Model file for the job. Use its own axes, mm. A direction names the side the tool comes from. Coordinates: 2 decimals unless noted, no trailing zeros. Write each loop counter-clockwise with the first axis right and the second up, starting at its lowest first coordinate (ties: lowest second). Pieces come first, ordered by that corner, then holes. Notation, with made-up numbers: M -37.5,-12 L -24.5,-12 A22 cw -24.5,25 Z; hole C 15,-16.5 d5. An arc over 180 degrees is marked long. Put each result on its own line as item: value. Start each with the question number.
Q1. Drill centre lines: line 1 along Y through (x, z) = (12.5, 4.7); line 2 along Y through (x, z) = (3.5, 5.55); line 3 along Z through (x, y) = (35.5, 0.25). Where is each one in solid material? Low to high.
Q2. Drop flat-ended pins along their axis: pin 1 (8 mm diameter, centred on x = 32, y = 2, fed in from -Z); pin 2 (3 mm diameter, centred on x = 4, y = 1.5, fed in from +Z). Give the stop position or say it passes through.
Q3. Cut at C-C (z = 2.25). Write the cut outline in (x, y), then the cut area to 3 significant figures.
Q4. Cut at B-B (x = 19). Write the cut outline in (y, z).
Q5. Which spindle directions (+Z, -Z, +X, -X, +Y, -Y) get a long thin tool onto all of the face, cutting with end or side? Do faces 1 (the cylindrical face through (19.783, 3.301, 0.285)), 2 (the cylindrical face through (0.301, 0.105, 0.285)), 3 (the flat face through (19, 6, 3)). Say none if no direction does.
Q6. Cut at D-D (y = 5.25). Write the cut outline in (x, z).
Q7. Pull direction Y, two halves, no side cores. Call faces 4 (the flat face through (19, 4, 1.5)), 5 (the cylindrical face through (19.874, -7.199, 0.285)), 6 (the flat face through (0, 0.5, 1.3)): pulls with the +Y half, pulls with the -Y half, needs draft (parallel to the pull), parting line crosses it, or undercut.
Q8. Cut at A-A (y = 0). Write the cut outline in (x, z), then the cut area to 3 significant figures.
```python
from build123d import *

# Parameters (mm, degrees)
PAD_DEPTH    = 39.2
SKETCH001_W  = 7
SKETCH001_H  = 24.2
POCKET_DEPTH = 6.001
FILLET_R     = 1


with BuildPart() as part:
    # Sketch → Pad (new body)
    with BuildSketch(Plane.YZ):
        Polygon((7.5, 0), (7.5, 6), (5.75, 6), (5.75, 5.25), (6, 5), (6, 1.5), (-6, 1.5), (-6, 5), (-5.75, 5.25), (-5.75, 6), (-7.5, 6), (-7.5, 0), align=None)
    extrude(amount=PAD_DEPTH)

    # Sketch001 (on Face12 of Pad) → Pocket (cut, through all)
    with BuildSketch(Plane.YX):
        with Locations((-0.5, 19.6)):
            Rectangle(SKETCH001_W, SKETCH001_H)
    extrude(amount=-POCKET_DEPTH, mode=Mode.SUBTRACT)

    # Fillet
    fillet_edges = [part.edges().sort_by_distance(p)[0] for p in [
        (19.6, -7.5, 0),
        (0, 0, 0),
        (39.2, 0, 0),
        (19.6, 7.5, 0),
        (19.6, -4, 0),
        (31.7, -0.5, 0),
        (19.6, 3, 0),
        (7.5, -0.5, 0),
    ]]
    fillet(fillet_edges, radius=FILLET_R)


solid = part.part
```
Computed values:
1. line 1: -7.5 to -6, 6 to 7.5
1. line 2: -7.5 to -5.75, 5.75 to 7.5
1. line 3: 0 to 1.5
2. pin 1: z = 0
2. pin 2: z = 1.5
3. outline: M 0,-7.5 L 39.2,-7.5 L 39.2,-6 L 0,-6 Z; M 0,6 L 39.2,6 L 39.2,7.5 L 0,7.5 Z
3. area: 118 mm2
4. outline: M -7.5,1 A1 ccw -6.5,0 L -5,0 A1 ccw -4,1 L -4,1.5 L -6,1.5 L -6,5 L -5.75,5.25 L -5.75,6 L -7.5,6 Z; M 3,1 A1 ccw 4,0 L 6.5,0 A1 ccw 7.5,1 L 7.5,6 L 5.75,6 L 5.75,5.25 L 6,5 L 6,1.5 L 3,1.5 Z
5. face 1: -Z
5. face 2: -Z, -X, +Y, -Y
5. face 3: +X, -X
6. outline: M 0,1 A1 ccw 1,0 L 38.2,0 A1 ccw 39.2,1 L 39.2,1.5 L 0,1.5 Z
7. face 4: undercut
7. face 5: pulls with the -Y half
7. face 6: needs draft
8. outline: M 0,1 A1 ccw 1,0 L 6.5,0 A1 ccw 7.5,1 L 7.5,1.5 L 0,1.5 Z; M 31.7,1 A1 ccw 32.7,0 L 38.2,0 A1 ccw 39.2,1 L 39.2,1.5 L 31.7,1.5 Z
8. area: 21.6 mm2
